Autodesk Inventor part; units mm, degrees
ref_plane "YZ Plane" through (0, 0, 0) normal (1, 0, 0) x (0, 1, 0)
ref_plane "XZ Plane" through (0, 0, 0) normal (0, 1, 0) x (-1, 0, 0)
ref_plane "XY Plane" through (0, 0, 0) normal (0, 0, 1) x (1, 0, 0)
sketch "Esboço1" plane through (0, 0, 0) normal (0, 1, 0) x (-1, 0, 0)
  line L0 (0, 0) -> (80, 0)
  line L1 (80, 0) -> (80, -80)
  line L2 (80, -80) -> (0, -80)
  line L3 (0, -80) -> (0, 0)
  dimension "d0" = 80
  dimension "d1" = 80
extrude "Extrusão1" add sketch "Esboço1" along normal blind 6
sketch "Esboço2" plane through (0, 6, 0) normal (0, 1, 0) x (1, 0, 0)
  line L0 (0, 80) -> (-80, 80)
  line L1 (-80, 80) -> (-80, 0)
  line L2 (-80, 0) -> (0, 0)
  line L3 (0, 0) -> (0, 80)
  point P0 (-8, 8)
  point P1 (-72, 8)
  point P2 (-72, 72)
  point P3 (-8, 72)
  dimension "d4" = 8
  dimension "d5" = 8
  dimension "d6" = 8
  dimension "d7" = 8
  dimension "d8" = 8
  dimension "d9" = 8
  dimension "d10" = 8
  dimension "d11" = 8
hole "Furo1" at (-8, 6, -8) at (-72, 6, -8) at (-72, 6, -72) at (-8, 6, -72) direction (0, -1, 0) diameter 5 depth 6
sketch "Esboço3" plane through (0, 6, 0) normal (0, 1, 0) x (1, 0, 0)
  line L0 (-80, 0) -> (0, 0)
  line L1 (-80, 80) -> (-80, 0)
  line L2 (0, 80) -> (-80, 80)
  line L3 (0, 0) -> (0, 80)
  point P0 (-40, 40)
  dimension "d19" = 80
  dimension "d20" = 40
  dimension "d21" = 40
hole "Furo2" at (-40, 6, -40) direction (0, -1, 0) diameter 15 depth 6
equation "\"d17\" = Espessura"
equation "\"Raio_vergadura\" = Espessura"
equation "\"Largura_alívio_de_vergadura\" = Espessura"
equation "\"Profundidade_alívio_de_vergadura\" = 0.5 * Espessura"
equation "\"Tamanho_alívio_de_dobra\" = 4 * Espessura"
equation "\"Remanescente_mínimo\" = 2 * Espessura"
equation "\"Raiodetransição\" = Raio_vergadura"
equation "\"Tamanho_de_raio_de_Jacobi\" = Raio_vergadura"
equation "\"TamanhoFolga\" = Espessura"
properties part number "Suporte inferior do eixo" material "Aluminum 6061"
Part model, mm, in its own coordinate system. Coordinates: 2 decimals unless noted, no trailing zeros. Order: outer loops, then holes, each group sorted by start corner. A loop starts at its lowest first (then second) coordinate and runs counter-clockwise, first axis right, second up.
(1) Slice it at C-C, the plane x = -8. Write the cut outline in (y, z).
Check sheet entries:
outline: (0, -80) - (6, -80) - (6, -74.5) - (0, -74.5) - close; (0, -69.5) - (6, -69.5) - (6, -10.5) - (0, -10.5) - close; (0, -5.5) - (6, -5.5) - (6, 0) - (0, 0) - close
(2) Pull direction Z, two halves, no side cores. Call faces 1 (the face through (-70.5, 3, -74)), 2 (the face through (0, 3, -41)), 3 (the face through (-39, 3, 0)): pulls with the +Z half, pulls with the -Z half, needs draft (parallel to the pull), parting line crosses it, or undercut.
Check sheet entries:
face 1: undercut
face 2: needs draft
face 3: pulls with the +Z half
(3) Slice it at D-D, the plane y = 5.05. Write the cut outline in (x, z).
Check sheet entries:
outline: (-80, -80) - (0, -80) - (0, 0) - (-80, 0) - close; hole circle Ø5 at (-72, -72); hole circle Ø5 at (-72, -8); hole circle Ø15 at (-40, -40); hole circle Ø5 at (-8, -72); hole circle Ø5 at (-8, -8)
(4) Slice it at A-A, the plane x = -40. Write the cut outline in (y, z).
Check sheet entries:
outline: (0, -80) - (6, -80) - (6, -47.5) - (0, -47.5) - close; (0, -32.5) - (6, -32.5) - (6, 0) - (0, 0) - close
(5) Probe L1, parallel to X at y = 4.6, z = -8; L2, parallel to X at y = 3.4, z = -40. List the from-to ranges inside material, lowest first.
Check sheet entries:
L1: x = -80 to -74.5, -69.5 to -10.5, -5.5 to 0
L2: x = -80 to -47.5, -32.5 to 0
(6) Slice it at B-B, the plane z = -8. Write the cut outline in (x, y), and give its area (3 significant figures).
Check sheet entries:
outline: (-80, 0) - (-74.5, 0) - (-74.5, 6) - (-80, 6) - close; (-69.5, 0) - (-10.5, 0) - (-10.5, 6) - (-69.5, 6) - close; (-5.5, 0) - (0, 0) - (0, 6) - (-5.5, 6) - close
area: 420 mm2
